Input: dimensioned drawing with shaded views. Units: mm. Origin: part minimum x, y, z. Give positions to 0.01 mm unless a question says otherwise; leave off trailing zeros. Loops run counter-clockwise (first coordinate to the right, second up) from the corner with the lowest first, then second, coordinate; pieces in that order, holes last. Notation, with made-up numbers: (-39, 34) -> (15, 34) arc R22 cw to (15, 67) -> close; hole circle Ø6 at (24, -0.75). An arc over 180 degrees is marked (long way). Answer in a Markdown table with one row per item. Add a question column.
1) Section query B-B (x = 100). Return the cut outline in (y, z).
2) Section query C-C (z = 34). Return the cut outline in (x, y).
3) First-contact query: P1, Ø1.5, axis at x = 66, z = 50, coming from the +Y side; P2, Ø4, axis at x = 56.5, z = 109.5, coming from the +Y side. Flat tips, straight axial feed; report the tip coordinate or a pass-through.
4) Section query A-A (y = 24). Return the cut outline in (x, z).
5) Section query D-D (x = 9.5). Return the cut outline in (y, z).
6) Line query: line 1 (Z direction, x = 32, y = 18.5); line 2 (Z direction, x = 49, y = 23.5); line 3 (Y direction, x = 51.5, z = 71.5). Output: solid intervals per line, ascending. Write a range as from..to.
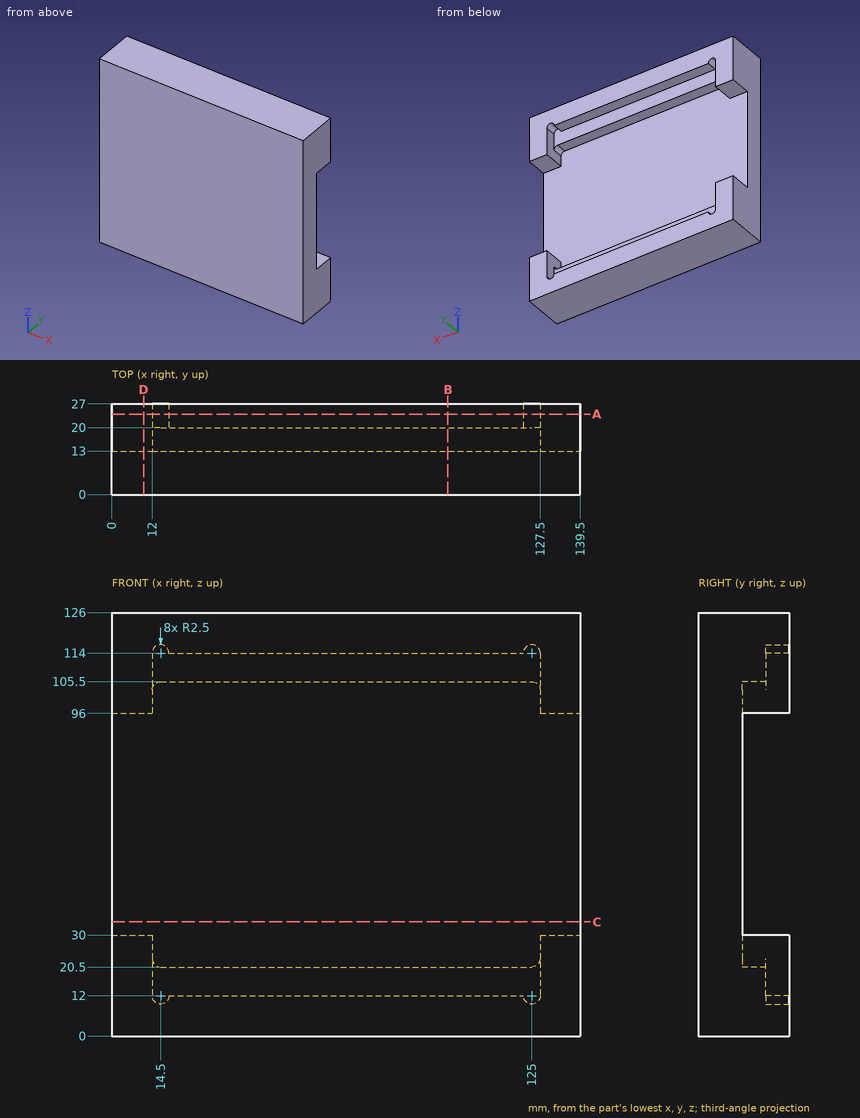
Evaluation:
| question | item | result |
|---|---|---|
| 1 | outline | (0, 0) -> (27, 0) -> (27, 12) -> (20, 12) -> (20, 20.5) -> (13, 20.5) -> (13, 105.5) -> (20, 105.5) -> (20, 114) -> (27, 114) -> (27, 126) -> (0, 126) -> close |
| 2 | outline | (0, 0) -> (139.5, 0) -> (139.5, 13) -> (0, 13) -> close |
| 3 | P1 | y = 13 |
| 3 | P2 | y = 20 |
| 4 | outline | (0, 0) -> (139.5, 0) -> (139.5, 30) -> (127.5, 30) -> (127.5, 12) arc R2.5 cw to (122.5, 12) -> (17, 12) arc R2.5 cw to (12, 12) -> (12, 30) -> (0, 30) -> close; (0, 96) -> (12, 96) -> (12, 114) arc R2.5 cw to (17, 114) -> (122.5, 114) arc R2.5 cw to (127.5, 114) -> (127.5, 96) -> (139.5, 96) -> (139.5, 126) -> (0, 126) -> close |
| 5 | outline | (0, 0) -> (27, 0) -> (27, 30) -> (13, 30) -> (13, 96) -> (27, 96) -> (27, 126) -> (0, 126) -> close |
| 6 | line 1 | 0..20.5, 105.5..126 |
| 6 | line 2 | 0..12, 114..126 |
| 6 | line 3 | 0..13 |
